Input: dimensioned drawing with shaded views. Units: mm. Origin: part minimum x, y, z. Coordinates: 2 decimals unless noted, no trailing zeros. Write each loop counter-clockwise with the first axis right and the second up, starting at its lowest first coordinate (ties: lowest second). Pieces come first, ordered by that corner, then holes. Notation, with made-up numbers: M -27,-23 L -16,-23 A33 ccw -16,6 Z; hole C 76,-26 d9. An arc over 180 degrees is marked long. Write each question's results on one line, items separated by ' | '. Start each with the question number.
1. First-contact query: pin 1 (2.5 mm diameter, centred on x = 67.5, y = 5, fed in from +Z). Flat tip, straight axial feed; report the tip coordinate or a pass-through.
2. Ray query, probe 1 along Y at (x, z) = (67.5, 0.95); probe 2 along X at (y, z) = (5.5, 1.05); probe 3 along X at (y, z) = (100, 1.4). Return the intervals inside material, ascending.
3. Section query A-A, the plane x = 90. Output: boundary loops of the cut face in (y, z).
4. Section query B-B, the plane y = 100. Output: boundary loops of the cut face in (x, z).
5. Section query C-C, the plane x = 47.5. Output: boundary loops of the cut face in (y, z), and give its area (3 significant figures).
6. Section query D-D, the plane y = 5. Output: boundary loops of the cut face in (x, z), and give its area (3 significant figures).
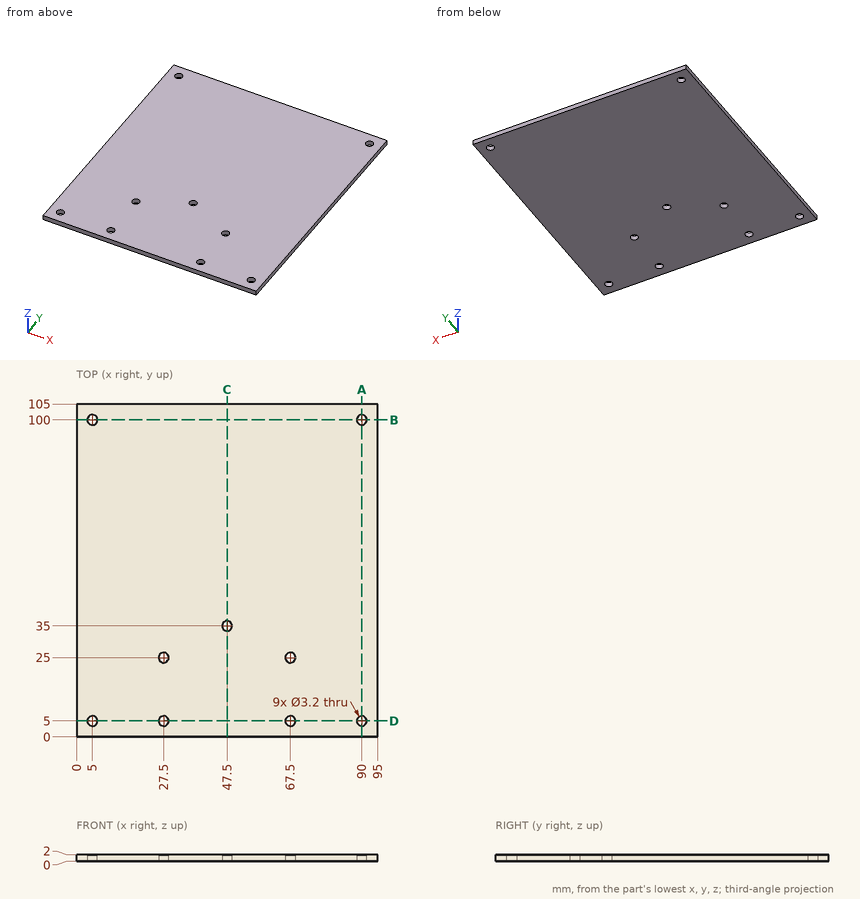
Answer:
1) pin 1: through
2) probe 1: 0 to 3.4, 6.6 to 23.4, 26.6 to 105 | probe 2: 0 to 3.48, 6.52 to 25.98, 29.02 to 65.98, 69.02 to 88.48, 91.52 to 95 | probe 3: 0 to 3.4, 6.6 to 88.4, 91.6 to 95
3) outline: M 0,0 L 3.4,0 L 3.4,2 L 0,2 Z; M 6.6,0 L 98.4,0 L 98.4,2 L 6.6,2 Z; M 101.6,0 L 105,0 L 105,2 L 101.6,2 Z
4) outline: M 0,0 L 3.4,0 L 3.4,2 L 0,2 Z; M 6.6,0 L 88.4,0 L 88.4,2 L 6.6,2 Z; M 91.6,0 L 95,0 L 95,2 L 91.6,2 Z
5) outline: M 0,0 L 33.4,0 L 33.4,2 L 0,2 Z; M 36.6,0 L 105,0 L 105,2 L 36.6,2 Z | area: 204 mm^2
6) outline: M 0,0 L 3.4,0 L 3.4,2 L 0,2 Z; M 6.6,0 L 25.9,0 L 25.9,2 L 6.6,2 Z; M 29.1,0 L 65.9,0 L 65.9,2 L 29.1,2 Z; M 69.1,0 L 88.4,0 L 88.4,2 L 69.1,2 Z; M 91.6,0 L 95,0 L 95,2 L 91.6,2 Z | area: 164 mm^2
